Check sheet for the modelled part. Datum: model origin and axes. Units: mm. A direction names the side the tool comes from. Round coordinates to 2 decimals unless told otherwise and drop trailing zeros. Order: outer loops, then holes, each group sorted by start corner. A loop starts at its lowest first (then second) coordinate and runs counter-clockwise, first axis right, second up.
(1) Tool access check on faces 5 (the flat face through (0, 10, 0)), 6 (the flat face through (-3, 0, 2)), 7 (the cylindrical face through (2.63, 16.07, -0.34)). Record the directions out of +Z, -Z, +X, -X, +Y, -Y that give a thin tool (end or side, any length) a straight path to the whole face; none if there is none.
(2) Sectioned sample at A-A, the plane x = 0. Enter the section's corners in (y, z), and give its area (3 significant figures).
(3) Mould release check, pull along Z, two halves, no side actions. Record for faces 1 (the flat face through (1, 21, -3)), 2 (the flat face through (0, 11, 0)), 3 (the cylindrical face through (2.7, 4.93, -1.72)), 4 (the cylindrical face through (3.905, 10.353, 0.867)): released by +Z, released by -Z, zero draft, split by the parting line, or undercut.
(4) Depth check by flat-ended pin: pin 1 (3 mm diameter, centred on x = -0.5, z = -1.5, fed in from -Y). Enter the tip coordinate at first touch or a pass-through.
(5) Sectioned sample at B-B, the plane y = 11.5. Enter the section's corners in (x, z), and give its area (3 significant figures).
(6) Thickness scan on probe 1 along X at (y, z) = (2, 0); probe 2 along Y at (x, z) = (-3.5, 0.75); probe 3 along Y at (x, z) = (1.75, 1.75). Record the ranges inside material, lowest first.
(7) Sectioned sample at D-D, the plane z = 3. Enter the section's corners in (x, y), and give its area (3 significant figures).
(8) Sectioned sample at C-C, the plane z = -2. Enter the section's corners in (x, y).
```python
from build123d import *

# Parameters (mm, degrees)
SKETCH1_R           = 4
BOSS_EXTRUDE1_DEPTH = 21
SKETCH2_R           = 3.2
CUT_EXTRUDE1_DEPTH  = 10
SKETCH3_R           = 2.65
CUT_EXTRUDE3_DEPTH  = 10


with BuildPart() as part:
    # Sketch1 → Boss-Extrude1 (new body)
    with BuildSketch(Plane(origin=(0, 0, 0), x_dir=(1, 0, 0), z_dir=(0, 1, 0))):
        with Locations(Location((0, 0, 0), (0, 0, 90))):
            Circle(SKETCH1_R)
    extrude(amount=BOSS_EXTRUDE1_DEPTH)

    # Sketch2 → Cut-Extrude1 (cut)
    with BuildSketch(Plane.XZ):
        with Locations(Location((0, 0, 0), (0, 0, 270))):
            Circle(SKETCH2_R)
    extrude(amount=-CUT_EXTRUDE1_DEPTH, mode=Mode.SUBTRACT)

    # Sketch3 → Cut-Extrude3 (cut)
    with BuildSketch(Plane(origin=(0, 21, 0), x_dir=(1, 0, 0), z_dir=(0, 1, 0))):
        with Locations(Location((0, 0, 0), (0, 0, 270))):
            Circle(SKETCH3_R)
    extrude(amount=-CUT_EXTRUDE3_DEPTH, mode=Mode.SUBTRACT)

    # Cut-Extrude5: read off the stored shape, not the designer's step
    # Cut-Extrude5: loft between two sections, ruled curve by curve
    cut_extrude5_from = [
        Edge.make_three_point_arc((-2.24981464, 14.6, 0), (-2.24981464, 16, 1.4), (-2.24981464, 17.4, 0)),
        Edge.make_three_point_arc((-2.24981464, 17.4, 0), (-2.24981464, 16, -1.4), (-2.24981464, 14.6, 0)),
    ]
    cut_extrude5_to = [
        Edge.make_three_point_arc((-3.999916451, 14.6, 0), (-3.999916451, 16, 1.4), (-3.999916451, 17.4, 0)),
        Edge.make_three_point_arc((-3.999916451, 17.4, 0), (-3.999916451, 16, -1.4), (-3.999916451, 14.6, 0)),
    ]
    cut_extrude5 = Solid(Shell([*[Face.make_surface_from_curves(cut_extrude5_from[k], cut_extrude5_to[k]) for k in range(2)], Face(Wire(cut_extrude5_from)), Face(Wire(cut_extrude5_to))]))
    add(cut_extrude5, mode=Mode.SUBTRACT)

    # Cut-Extrude5 2: loft between two sections, ruled curve by curve
    cut_extrude5_2_from = [
        Edge.make_three_point_arc((-2.877351837, 3.6, 0), (-2.877351837, 5, 1.4), (-2.877351837, 6.4, 0)),
        Edge.make_three_point_arc((-2.877351837, 6.4, 0), (-2.877351837, 5, -1.4), (-2.877351837, 3.6, 0)),
    ]
    cut_extrude5_2_to = [
        Edge.make_three_point_arc((-3.999916451, 3.6, 0), (-3.999916451, 5, 1.4), (-3.999916451, 6.4, 0)),
        Edge.make_three_point_arc((-3.999916451, 6.4, 0), (-3.999916451, 5, -1.4), (-3.999916451, 3.6, 0)),
    ]
    cut_extrude5_2 = Solid(Shell([*[Face.make_surface_from_curves(cut_extrude5_2_from[k], cut_extrude5_2_to[k]) for k in range(2)], Face(Wire(cut_extrude5_2_from)), Face(Wire(cut_extrude5_2_to))]))
    add(cut_extrude5_2, mode=Mode.SUBTRACT)


solid = part.part
```
Derived:
1. face 5: -Y
1. face 6: +Z, -Z, +X, -X, -Y
1. face 7: +Y
2. outline: (0, -4) - (21, -4) - (21, -2.65) - (11, -2.65) - (11, 2.65) - (21, 2.65) - (21, 4) - (0, 4) - (0, 3.2) - (10, 3.2) - (10, -3.2) - (0, -3.2) - close
2. area: 51.0 mm2
3. face 1: zero draft
3. face 2: undercut
3. face 3: undercut
3. face 4: split by the parting line
4. pin 1: stops at y = 10
5. outline: circle Ø8 at (0, 0); hole circle Ø5.3 at (0, 0)
5. area: 28.2 mm2
6. probe 1: x = -4 to -3.2, 3.2 to 4
6. probe 2: y = 0 to 3.82, 6.18 to 14.82, 17.18 to 21
6. probe 3: y = 10 to 11
7. outline: (-2.65, 0) - (-1.11, 0) - (-1.11, 10) - (1.11, 10) - (1.11, 0) - (2.65, 0) - (2.65, 21) - (-2.65, 21) - close
7. area: 88.9 mm2
8. outline: (-3.46, 0) - (-2.5, 0) - (-2.5, 10) - (2.5, 10) - (2.5, 0) - (3.46, 0) - (3.46, 21) - (1.74, 21) - (1.74, 11) - (-1.74, 11) - (-1.74, 21) - (-3.46, 21) - close
